Source: CAD feature listing. Evaluate the final solid. Frame: model axes, mm. A direction names the side the tool comes from. Coordinates: 2 decimals unless noted, no trailing zeros. Write each loop counter-clockwise with the first axis right and the second up, starting at its lowest first coordinate (ties: lowest second). Pieces come first, ordered by that corner, then holes. Notation, with made-up numbers: (74, -6) -> (118, -6) arc R18 cw to (118, 14) -> close; hole circle Ø3 at (60.25, 10). An arc over 180 degrees is marked (long way). Write item = value, one per line.
Autodesk Inventor part; units mm, degrees
ref_plane "YZ Plane" through (0, 0, 0) normal (1, 0, 0) x (0, 1, 0)
ref_plane "XZ Plane" through (0, 0, 0) normal (0, 1, 0) x (-1, 0, 0)
ref_plane "XY Plane" through (0, 0, 0) normal (0, 0, 1) x (1, 0, 0)
sketch "Sketch1" plane through (0, 0, 0) normal (0, 0, 1) x (1, 0, 0)
  line L0 (0, 0) -> (-56.9976, 0)
  line L1 (-56.9976, 0) -> (-56.9976, 12.7)
  line L2 (-56.9976, 12.7) -> (0, 12.7)
  line L3 (0, 12.7) -> (0, 0)
  line L4 (0, 12.7) -> (-7.493, 12.7)
  line L5 (-7.493, 12.7) -> (-7.493, 6.35)
  line L6 (-56.9976, 12.7) -> (-49.5046, 12.7)
  line L7 (-49.5046, 12.7) -> (-49.5046, 6.35)
  circle A0 centre (-49.5046, 6.35) radius 3.302
  circle A1 centre (-7.493, 6.35) radius 3.302
  dimension "d1" = 56.9976
  dimension "d2" = 12.7
  dimension "d3" = 7.493
  dimension "d4" = 6.35
  dimension "d5" = 7.493
  dimension "d6" = 6.604
  dimension "d7" = 6.604
  dimension "d19" = 6.35
extrude "Plate1" add sketch "Sketch1" along normal blind 3.175
sketch "Sketch3" plane through (9.525, 0, -9.525) normal (1, 0, 0) x (0, 1, 0)
  line L0 (12.7, 0) -> (0, 0)
  line L1 (0, 0) -> (0, -208.2038)
  line L2 (0, -208.2038) -> (12.7, -208.2038)
  line L3 (12.7, -208.2038) -> (12.7, 0)
edge flange "Flange2" height 220.9038 angle 90 thickness 3.175 bend radius 9.525 thickness toward (1, 0, 0) relief tear relief width 3.175 relief depth 1.5875 edges at (0, 6.35, 0) wall of the first edge with corners at (9.525, 12.7, -9.525) (9.525, 0, -9.525) (9.525, 0, -217.7288) (9.525, 12.7, -217.7288)
bend "Bend2"
corner "Corner2"
sketch "Sketch4" plane through (0, 0, -227.2538) normal (0, 0, -1) x (-1, 0, 0)
  line L0 (0, 12.7) -> (0, 0)
  line L1 (0, 0) -> (50.6476, 0)
  line L2 (50.6476, 0) -> (50.6476, 12.7)
  line L3 (50.6476, 12.7) -> (0, 12.7)
edge flange "Flange3" height 63.3476 angle 90 thickness 3.175 bend radius 9.525 thickness toward (0, 0, -1) relief tear relief width 3.175 relief depth 1.5875 edges at (9.525, 6.35, -217.7288) wall of the first edge with corners at (0, 12.7, -227.2538) (0, 0, -227.2538) (-50.6476, 0, -227.2538) (-50.6476, 12.7, -227.2538)
bend "Bend3"
corner "Corner3"
sketch "Sketch5" plane through (0, 0, 3.175) normal (0, 0, 1) x (1, 0, 0)
  circle A0 centre (-7.493, 6.35) radius 3.302
  circle A1 centre (-49.5046, 6.35) radius 3.302
extrude "Extrusion1" cut sketch "Sketch5" against normal blind 2286
equation "\"d20\" = BendReliefWidth"
equation "\"d21\" = BendReliefDepth"
equation "\"d22\" = MinimumRemnant"
equation "\"d23\" = BendRadius"
equation "\"d27\" = CornerReliefSize"
equation "\"d28\" = GapSize"
equation "\"d29\" = JacobiRadiusSize"
equation "\"d30\" = BendReliefWidth"
equation "\"d31\" = BendReliefDepth"
equation "\"d32\" = MinimumRemnant"
equation "\"d33\" = BendRadius"
equation "\"d37\" = CornerReliefSize"
equation "\"d38\" = GapSize"
equation "\"d39\" = JacobiRadiusSize"
equation "\"BendRadius\" = Thickness"
equation "\"BendReliefWidth\" = Thickness"
equation "\"BendReliefDepth\" = 0.5 * Thickness"
equation "\"CornerReliefSize\" = 4 * Thickness"
equation "\"MinimumRemnant\" = 2 * Thickness"
equation "\"TransitionRadius\" = BendRadius"
equation "\"JacobiRadiusSize\" = BendRadius"
equation "\"GapSize\" = Thickness"
equation "\"d8\" = BendRadius"
properties part number "tie-together tier 1" material "Aluminum 6061"
1) Pull-direction query (Z, two-part tool) for faces 1 (the flat face through (-29, 6, 0)), 2 (the cylindrical face through (-46.204, 6.261, -228.819)), 3 (the flat face through (-29, 6, 3.175)); classes: +Z half, -Z half, draft (parallel to the pull), parting line (faces both ways), or undercut.
Answer block:
face_1 = undercut
face_2 = draft
face_3 = +Z half
2) First-contact query: pin 1 Ø3.5 at (y, z) = (1, -229) entering from -X; pin 2 Ø4 at (x, y) = (-49.5, 6.35) entering from -Z; pin 3 Ø2 at (y, z) = (3.5, -119) entering from -X (3 decimals). Flat tips, straight axial feed; report the tip coordinate or a pass-through.
Answer block:
pin_1 = -50.65
pin_2 = through
pin_3 = 9.525
3) Cut plane B-B, the plane x = -20. Output: boundary loops of the cut face in (y, z) (3 decimals).
Answer block:
outline = (0, -230.429) -> (12.7, -230.429) -> (12.7, -227.254) -> (0, -227.254) -> close; (0, 0) -> (12.7, 0) -> (12.7, 3.175) -> (0, 3.175) -> close
4) Cut plane C-C, the plane z = -149. Output: boundary loops of the cut face in (x, y) (3 decimals), and give its area (3 significant figures).
Answer block:
outline = (9.525, 0) -> (12.7, 0) -> (12.7, 12.7) -> (9.525, 12.7) -> close
area = 40.3 mm2
5) Material intervals for probe 1 along Z at (x, y) = (-3, 10.75) (3 decimals); probe 2 along X at (y, z) = (3.25, -166) (3 decimals); probe 3 along X at (y, z) = (6.35, 1.9) (3 decimals), sorted ascending. Write a range as [from, to].
Answer block:
probe_1 = [-230.429, -227.254], [0, 3.175]
probe_2 = [9.525, 12.7]
probe_3 = [-56.998, -52.807], [-46.203, -10.795], [-4.191, 5.546]
6) Reachability of faces 4 (the cylindrical face through (6.7, 6.3, -224.5)), 5 (the flat face through (11, 0, -114)) from +Z, -Z, +X, -X, +Y, -Y: full face, straight path, thin tool, end or side. Return the list, or none.
Answer block:
face_4 = -X, +Y, -Y
face_5 = +Z, -Z, +X, -X, -Y
7) Cut plane D-D, the plane x = 7.5. Output: boundary loops of the cut face in (y, z).
Answer block:
outline = (0, -227.98) -> (12.7, -227.98) -> (12.7, -223.6) -> (0, -223.6) -> close; (0, -3.65) -> (12.7, -3.65) -> (12.7, 0.72) -> (0, 0.72) -> close
8) Cut plane A-A, the plane y = 6.35. Output: boundary loops of the cut face in (x, z) (3 decimals), and give its area (3 significant figures).
Answer block:
outline = (-56.998, 0) -> (-52.807, 0) -> (-52.807, 3.175) -> (-56.998, 3.175) -> close; (-46.203, -230.429) -> (-10.795, -230.429) -> (-10.795, -227.254) -> (-46.203, -227.254) -> close; (-46.203, 0) -> (-10.795, 0) -> (-10.795, 3.175) -> (-46.203, 3.175) -> close; (-4.191, -230.429) -> (0, -230.429) arc R12.7 ccw to (12.7, -217.729) -> (12.7, -9.525) arc R12.7 ccw to (0, 3.175) -> (-4.191, 3.175) -> (-4.191, 0) -> (0, 0) arc R9.525 cw to (9.525, -9.525) -> (9.525, -217.729) arc R9.525 cw to (0, -227.254) -> (-4.191, -227.254) -> close
area = 1,040 mm2
